from build123d import *

# Parameters (mm, degrees)
PAD_DEPTH            = 10
THICKNESS_T          = -2
PAD001_DEPTH         = 18
SKETCH002_R          = 5.5
SKETCH002_R_2        = 3.5
PAD002_DEPTH         = 8
SKETCH003_W          = 33.990382
SKETCH003_H          = 16.5
PAD003_DEPTH         = 2
BODY_PLACEMENT_ANGLE = 134.999996


with BuildPart() as part:
    # Sketch → Pad (new body)
    with BuildSketch(Plane.YZ):
        with BuildLine():
            ThreePointArc((6.495191, 8.25), (-3.173595, 10.008911), (-10.062306, 3))
            Line((-10.062306, 3), (-10.062306, -3))
            ThreePointArc((-10.062306, -3), (-3.173595, -10.008911), (6.495191, -8.25))
            Line((6.495191, -8.25), (16.995191, -8.25))
            Line((16.995191, -8.25), (16.995191, 8.25))
            Line((16.995191, 8.25), (6.495191, 8.25))
        make_face()
    extrude(amount=PAD_DEPTH)

    # Thickness
    thickness_openings = [part.faces().sort_by_distance(p)[0] for p in [
        (10, 3.557762, 0),
    ]]
    offset(amount=THICKNESS_T, openings=thickness_openings)

    # Sketch001 → Pad001 (join)
    with BuildSketch(Plane.YZ):
        Polygon((16.995191, 8.25), (9.995191, 8.25), (9.995191, 3.75), (11.995191, 3.75), (11.995191, 6.25), (14.995191, 6.25), (14.995191, -6.249983), (11.995191, -6.25), (11.995191, -3.75), (9.995191, -3.75), (9.995191, -8.25), (16.995191, -8.25), align=None)
    extrude(amount=PAD001_DEPTH)

    # Sketch002 (on Face22 of Pad001) → Pad002 (join)
    with BuildSketch(Plane.YZ.offset(2)):
        Circle(SKETCH002_R)
        Circle(SKETCH002_R_2, mode=Mode.SUBTRACT)
    extrude(amount=PAD002_DEPTH)

    # Sketch003 → Pad003 (join)
    with BuildSketch(Plane.YZ):
        Rectangle(SKETCH003_W, SKETCH003_H)
    extrude(amount=PAD003_DEPTH)


with BuildPart() as part_1:
    # Body placement: moved
    add(part.part.moved(Location((0, -24.041634, 2.828429))).rotate(Axis((0, -24.041634, 2.828429), (1, 0, 0)), BODY_PLACEMENT_ANGLE))


solid = part_1.part
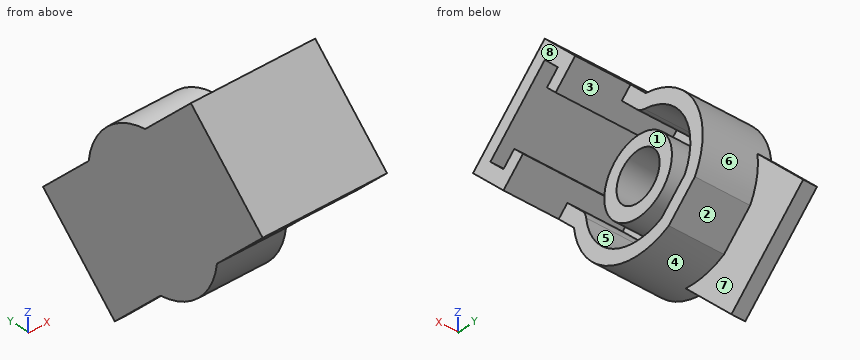
Build history of the part. All positions in model axes, mm. Face numbers are marked on the shaded views. A direction names the side the tool comes from. Coordinates: 2 decimals unless noted, no trailing zeros. Order: outer loops, then holes, each group sorted by start corner. A loop starts at its lowest first (then second) coordinate and runs counter-clockwise, first axis right, second up. Notation, with made-up numbers: (89, 28.5) - (121, 28.5) arc R21 ccw to (121, 54.5) - close; hole circle Ø5 at (20.25, 27). An arc over 180 degrees is marked (long way). Write each question's results on one line, items separated by ' | '. Start each with the question number.
Item 1: Mould opens along Y. For the marked faces 1, 2 and 3 say: released by +Y, released by -Y, zero draft, split by the parting line, or undercut.
Item 2: Band-saw the part on A-A on x = 4.5. Write the cut outline in (y, z) (1 decimal), and give its area (3 significant figures).
Item 3: Band-saw the part on D-D on x = 15.75. Write the cut outline in (y, z), and give its area (3 significant figures).
Item 4: Flat gauge pins, fed straight in: pin 1 (3.5 mm diameter, centred on y = -24.5, z = 4, fed in from +X); pin 2 (2 mm diameter, centred on x = 2.5, y = -22, fed in from +Z); pin 3 (10 mm diameter, centred on x = 10, z = 13.5, fed in from +Y). Where does each tip first touch, or does it go through?
Item 5: Band-saw the part on C-C on y = -37.5. Write the cut outline in (x, z), and give its area (3 significant figures).
Item 6: Wall check: probe 1 along Z at (x, y) = (5.5, -25); probe 2 along Y at (x, z) = (3.5, 2); probe 3 along Y at (x, z) = (5.5, -2). Give the ranges that are in metal, low to high. Write a range as [from, to].
Item 7: Tool access for the marked faces 4, 5, 6, 7 and 8: list every direction of +Z, -Z, +X, -X, +Y, -Y with a clear straight run to the whole face (end or side of a thin tool).
Item 8: Band-saw the part on B-B on z = 0.5. Write the cut outline in (x, y).
Numbers:
1) face 1: zero draft | face 2: released by +Y | face 3: undercut
2) outline: (-41.9, 9) - (-34.5, 1.6) arc R10.5 ccw to (-19, -6.4) - (-14.8, -2.2) arc R10.5 ccw to (-22.8, 13.3) - (-30.2, 20.7) - close; circle Ø11 at (-24, 2.8); hole (-39.1, 9) - (-36.9, 6.9) - (-35.2, 8.7) - (-33.8, 7.2) - (-35.5, 5.5) - (-33.1, 3) arc R2 cw to (-32.5, 1.8) arc R8.5 ccw to (-20.2, -4.8) - (-16.4, -1) arc R8.5 ccw to (-23, 11.3) arc R2 cw to (-24.2, 11.8) - (-26.7, 14.3) - (-28.5, 12.5) - (-29.9, 14) - (-28.1, 15.7) - (-30.2, 17.9) - close; hole circle Ø7 at (-24, 2.8) | area: 221 mm^2
3) outline: (-41.89, 9.01) - (-36.94, 4.06) - (-33.76, 7.24) - (-35.18, 8.66) - (-36.94, 6.89) - (-39.06, 9.01) - (-30.23, 17.85) - (-28.1, 15.73) - (-29.87, 13.96) - (-28.46, 12.55) - (-25.28, 15.73) - (-30.23, 20.68) - close | area: 63.0 mm^2
4) pin 1: x = 2 | pin 2: z = 13.45 | pin 3: y = -15.21
5) outline: (0, 4.62) - (18, 4.62) - (18, 7.45) - (2, 7.45) - (2, 10.58) - (18, 10.58) - (18, 13.4) - (0, 13.4) - close | area: 108 mm^2
6) probe 1: [-7.63, -5.62], [-2.59, -0.54], [6.19, 8.24], [12.63, 15.45] | probe 2: [-34.88, -32.51], [-29.48, -27.44], [-20.64, -18.6], [-15.58, -13.57] | probe 3: [-33.37, -31.04], [-26.68, -21.41], [-17.47, -14.72]
7) face 4: -Z, +X | face 5: +X | face 6: +X, +Y | face 7: -Z, +X, +Y | face 8: +Z, -Z, +X, +Y, -Y
8) outline: (0, -34.28) - (10, -34.28) - (10, -32.22) - (2, -32.22) - (2, -29.02) - (10, -29.02) - (10, -26.65) - (2, -26.65) - (2, -21.43) - (10, -21.43) - (10, -19.06) - (2, -19.06) - (2, -15.87) - (10, -15.87) - (10, -13.8) - (2, -13.8) - (2, -10.05) - (0, -10.05) - close
